Autodesk Inventor part; units mm, degrees
ref_plane "YZ Plane" through (0, 0, 0) normal (1, 0, 0) x (0, 1, 0)
ref_plane "XZ Plane" through (0, 0, 0) normal (0, 1, 0) x (-1, 0, 0)
ref_plane "XY Plane" through (0, 0, 0) normal (0, 0, 1) x (1, 0, 0)
sketch "Sketch1" plane through (0, 0, 0) normal (0, 0, 1) x (1, 0, 0)
  circle A0 centre (0, 0) radius 4
  dimension "Diameter" = 8
extrude "Extrusion1" add sketch "Sketch1" along normal blind 150
sketch "Sketch2" plane through (0, 0, 150) normal (0, 0, 1) x (1, 0, 0)
  circle A0 centre (0, 0) radius 4
  circle A1 centre (0, 0) radius 6.5
  dimension "Head_Diameter" = 13
extrude "Extrusion2" add sketch "Sketch2" along normal blind 8 contours A0 | A1
sketch "Sketch3" plane through (0, 0, 158) normal (0, 0, 1) x (1, 0, 0)
  circle A0 centre (0, 0) radius 6.5
  circle A1 centre (0, 0) radius 3.4641 construction
  line L0 (0, 3.4641) -> (3, 1.7321)
  line L1 (3, -1.7321) -> (3, 1.7321)
  line L2 (0, 3.4641) -> (-3, 1.7321)
  line L3 (-3, -1.7321) -> (-3, 1.7321)
  line L4 (-3, -1.7321) -> (0, -3.4641)
  line L5 (3, -1.7321) -> (0, -3.4641)
  dimension "Hex_Width" = 6
extrude "Extrusion3" cut sketch "Sketch3" against normal blind 4 contours L0 L1 L5 L4 L3 L2
thread "Thread1"
chamfer "Chamfer1" distance 0.8 angle 45 2 edges at (-6.5, 0, 158) (-4, 0, 0)
equation "\"d9\" = ThreadLength"
equation "\"d12\" = Chamfer"
equation "\"ThreadLength\" = 28"
properties part number "SCREW, SOC HD, P, 12.9, M8X1.25X150MM" material "Steel, MS"
Input: part model. Units: mm. Frame: model coordinates. A direction names the side the tool comes from. Give positions to 0.01 mm unless a question says otherwise; leave off trailing zeros. Loops run counter-clockwise (first coordinate to the right, second up) from the corner with the lowest first, then second, coordinate; pieces in that order, holes last. Notation, with made-up numbers: (41.5, 61) -> (65.5, 61) arc R25 ccw to (65.5, 83) -> close; hole circle Ø8 at (0.25, 83). An arc over 180 degrees is marked (long way). Use a Markdown table: item, result.
Q1. Access query for faces 4 (the flat face through (3, 0, 156)), 5 (the flat face through (3, 3, 150)), 6 (the flat face through (0, 0, 0)). Directions: +Z, -Z, +X, -X, +Y, -Y. A direction counts if a zero-diameter tool reaches every point of the face in a straight line with its end or side. Return the directions, or none.
Entries:
| item | result |
|---|---|
| face 4 | +Z |
| face 5 | -Z |
| face 6 | -Z, +X, -X, +Y, -Y |
Q2. Section query B-B, the plane z = 24. Return the cut outline in (x, y), plus the area to 3 significant figures.
Entries:
| item | result |
|---|---|
| outline | circle Ø8 at (0, 0) |
| area | 50.3 mm² |
Q3. Pull-direction query (X, two-part tool) for faces 1 (the flat face through (1.5, 2.6, 156)), 2 (the flat face through (2.5, -2.5, 158)), 3 (the cylindrical face through (-0.867, 3.905, 74.356)); classes: pulls with the +X half, pulls with the -X half, needs draft (parallel to the pull), parting line crosses it, or undercut.
Entries:
| item | result |
|---|---|
| face 1 | undercut |
| face 2 | needs draft |
| face 3 | parting line crosses it |
Q4. First-contact query: P1, Ø5, axis at x = 0, y = 1.5, coming from the -Z side; P2, Ø1.5, axis at x = -1, z = 44, coming from the +Y side; P3, Ø6, axis at y = 3.5, z = 82, coming from the -X side; P4, Ø3, axis at x = -0.5, y = 0, coming from the +Z side. Flat tips, straight axial feed; report the tip coordinate or a pass-through.
Entries:
| item | result |
|---|---|
| P1 | stops at z = 0 |
| P2 | stops at y = 3.99 |
| P3 | stops at x = -3.97 |
| P4 | stops at z = 154 |
Q5. Section query A-A, the plane y = 0. Return the cut outline in (x, z), plus the area to 3 significant figures.
Entries:
| item | result |
|---|---|
| outline | (-6.5, 150) -> (-4, 150) -> (-4, 0.8) -> (-3.2, 0) -> (3.2, 0) -> (4, 0.8) -> (4, 150) -> (6.5, 150) -> (6.5, 157.2) -> (5.7, 158) -> (3, 158) -> (3, 154) -> (-3, 154) -> (-3, 158) -> (-5.7, 158) -> (-6.5, 157.2) -> close |
| area | 1,280 mm² |
Q6. Ray query, probe 1 along Z at (x, y) = (5.25, -0.25); probe 2 along Z at (x, y) = (-1.25, 1); probe 3 along Y at (x, z) = (-0.25, 121). Return the intervals inside material, ascending. Write a range as from..to.
Entries:
| item | result |
|---|---|
| probe 1 | z = 150..158 |
| probe 2 | z = 0..154 |
| probe 3 | y = -3.99..3.99 |
